```python
from build123d import *

# Parameters (mm, degrees)
F_01_START                           = -7.23
S01_SMOOTH_PIN_AND_END_MARGIN_R      = 2.5
F_01_SMOOTH_PIN_AND_END_MARGIN_DEPTH = 16.67
F_02_START                           = -9.25
S02_CLEVIS_PIN_HEAD_R                = 4.15
F_02_CLEVIS_PIN_HEAD_DEPTH           = 2.02
F_03_START                           = 7.45
S03_DE_4_RETAINING_GROOVE_R          = 2.6
S03_DE_4_RETAINING_GROOVE_R_2        = 1.99
F_03_DE_4_RETAINING_GROOVE_DEPTH     = 0.75


with BuildPart() as part:
    # S01 - Smooth pin and end margin → 01 - Smooth pin and end margin (new body)
    with BuildSketch(Plane.XY.offset(F_01_START)):
        Circle(S01_SMOOTH_PIN_AND_END_MARGIN_R)
    extrude(amount=F_01_SMOOTH_PIN_AND_END_MARGIN_DEPTH)

    # S02 - Clevis pin head → 02 - Clevis pin head (add)
    with BuildSketch(Plane.XY.offset(F_02_START)):
        Circle(S02_CLEVIS_PIN_HEAD_R)
    extrude(amount=F_02_CLEVIS_PIN_HEAD_DEPTH)

    # S03 - DE-4 retaining groove → 03 - DE-4 retaining groove (cut)
    with BuildSketch(Plane.XY.offset(F_03_START)):
        Circle(S03_DE_4_RETAINING_GROOVE_R)
        Circle(S03_DE_4_RETAINING_GROOVE_R_2, mode=Mode.SUBTRACT)
    extrude(amount=F_03_DE_4_RETAINING_GROOVE_DEPTH, mode=Mode.SUBTRACT)


solid = part.part
```
Geometry check sheet. Reference: the model listing, model coordinates, mm. A direction names the side the tool comes from. Give positions to 0.01 mm unless a question says otherwise; leave off trailing zeros. Order: outer loops, then holes, each group sorted by start corner. A loop starts at its lowest first (then second) coordinate and runs counter-clockwise, first axis right, second up. Notation, with made-up numbers: (51.5, 1) -> (86.5, 1) arc R16 cw to (86.5, 31) -> close; hole circle Ø9 at (38.25, 40.25). An arc over 180 degrees is marked (long way). Write each question's results on one line, items separated by ' | '. Start each with the question number.
(1) Access from +Z, -Z, +X, -X, +Y, -Y to the whole of each face (thin tool, end or side, straight path). Record for faces 4 (the face through (-0.54, -2.44, 0.01)), 5 (the face through (-0.9, -4.05, -8.25)), 6 (the face through (-2, -1, 8.2)).
(2) Mould release check, pull along Z, two halves, no side actions. Record for faces 1 (the face through (2, -2, -7.23)), 2 (the face through (-0.259, 1.973, 7.82)), 3 (the face through (-0.54, -2.44, 8.81)): pulls with the +Z half, pulls with the -Z half, needs draft (parallel to the pull), parting line crosses it, or undercut.
(3) Scan lines: line 1 (Z direction, x = -1.75, y = -1.5); line 2 (Z direction, x = 2.25, y = 2.5); line 3 (X direction, y = -1, z = 6.5). Record each from-to range of solid material in increasing order.
(4) Sectioned sample at A-A (x = 0). Enter the section's corners in (y, z).
(5) Sectioned sample at C-C (z = -2.5). Enter the section's corners in (x, y), plus the area to 3 significant figures.
(6) Gauge pin test, flat ends, axial feed: P1, Ø4, axis at y = 2.5, z = -0.5, coming from the +X side; P2, Ø1, axis at y = -1, z = 6.5, coming from the -X side; P3, Ø3, axis at y = -1, z = 4, coming from the +X side. Record the tip position at first contact, or that the pin passes through.
(7) Sectioned sample at D-D (z = -7.5). Enter the section's corners in (x, y), plus the area to 3 significant figures.
Answer below:
1) face 4: +Z | face 5: +Z, -Z | face 6: none
2) face 1: pulls with the +Z half | face 2: undercut | face 3: needs draft
3) line 1: -9.25 to 7.45, 8.2 to 9.44 | line 2: -9.25 to -7.23 | line 3: -2.29 to 2.29
4) outline: (-4.15, -9.25) -> (4.15, -9.25) -> (4.15, -7.23) -> (2.5, -7.23) -> (2.5, 7.45) -> (1.99, 7.45) -> (1.99, 8.2) -> (2.5, 8.2) -> (2.5, 9.44) -> (-2.5, 9.44) -> (-2.5, 8.2) -> (-1.99, 8.2) -> (-1.99, 7.45) -> (-2.5, 7.45) -> (-2.5, -7.23) -> (-4.15, -7.23) -> close
5) outline: circle Ø5 at (0, 0) | area: 19.6 mm2
6) P1: x = 2.45 | P2: x = -2.45 | P3: x = 2.5
7) outline: circle Ø8.3 at (0, 0) | area: 54.1 mm2
